Design review of the part built by this model. Coordinates are the model's own, in mm. Face numbers are marked on the shaded views. Coordinates: 2 decimals unless noted, no trailing zeros. Order: outer loops, then holes, each group sorted by start corner. A loop starts at its lowest first (then second) coordinate and runs counter-clockwise, first axis right, second up. Notation, with made-up numbers: M -16.5,12 L 6.5,12 A14 ccw 6.5,22 Z; hole C 67,6.5 d5. An arc over 180 degrees is marked long. Answer as a JSON object with one key per item and string values.
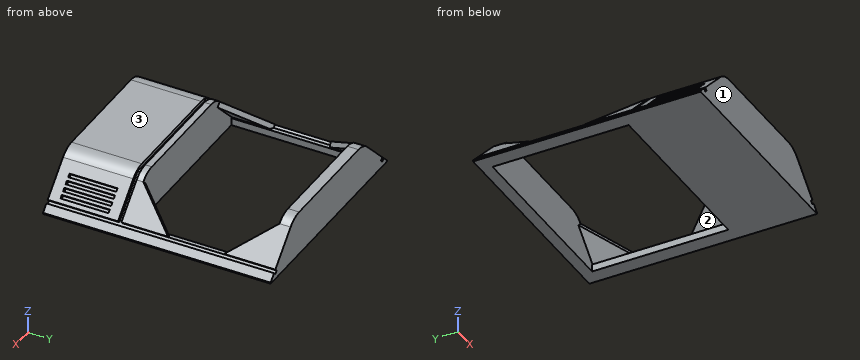
from build123d import *

# Parameters (mm, degrees)
F1_DEPTH  = 20.4
F3_DEPTH  = 0.3
F4_W      = 12.2
F4_H      = 3.3343145751
F5_DEPTH  = 8.8731825407
F6_W      = 8.2600505063
F6_H      = 12.2
F7_DEPTH  = 25
F8_W      = 4.3
F8_H      = 0.3
F9_DEPTH  = 0.3
F10_F1_R  = 2
F10_F2_R  = 2
F12_DEPTH = 0.5
F13_W     = 8.8721825407
F13_H     = 0.3
F14_DEPTH = 0.3
F16_DEPTH = 0.1


# Not quite as in the source:
# - a feature names something its author has since deleted; it is built from what else it names


with BuildPart() as f1:
    # F0 (on Front) → F1 (new body)
    with BuildSketch(Plane.XZ):
        Polygon((-9.65, 0), (0, 0), (0, 3.9), (-5.75, 3.9), align=None)
    extrude(amount=F1_DEPTH)

    # F2 (on face) → F3 (cut)
    with BuildSketch(Plane(origin=(-4.825, 0, 4.825), x_dir=(0, -1, 0), z_dir=(-0.7071067812, 0, 0.7071067812))):
        Polygon((13.8, -5.7235804385), (0, -5.7235804385), (0, -6.0235804385), (20.4, -6.0235804385), (20.4, -5.7235804385), (14.1, -5.7235804385), (14.1, 0.1956567054), (13.8, 0.1956567054), align=None)
    extrude(amount=-F3_DEPTH, mode=Mode.SUBTRACT)

    # F4 (on face) → F5 (cut, through all)
    with BuildSketch(Plane.YZ):
        with Locations((-7.1, 2.2328427125)):
            Rectangle(F4_W, F4_H)
    extrude(amount=-F5_DEPTH, mode=Mode.SUBTRACT)

    # F6 (on face) → F7 (cut)
    with BuildSketch(Plane.XY.offset(0.5656854249)):
        with Locations((-4.1300252532, -7.1)):
            Rectangle(F6_W, F6_H)
    extrude(amount=-F7_DEPTH, mode=Mode.SUBTRACT)

    # F8 (on face) → F9 (cut)
    with BuildSketch(Plane(origin=(-4.825, 0, 4.825), x_dir=(0, -1, 0), z_dir=(-0.7071067812, 0, 0.7071067812))):
        with Locations((17.25, -3.3735804385)):
            Rectangle(F8_W, F8_H)
        with Locations((17.25, -3.9735804385)):
            Rectangle(F8_W, F8_H)
        with Locations((17.25, -5.1735804385)):
            Rectangle(F8_W, F8_H)
        with Locations((17.25, -4.5735804385)):
            Rectangle(F8_W, F8_H)
    extrude(amount=-F9_DEPTH, mode=Mode.SUBTRACT)

    # F10: fillet of radius 2 on 3 edges, made by hand

    # F10_f1
    f10_f1_edges = [f1.edges().sort_by_distance(p)[0] for p in [
        (-5.75, -0.5, 3.9),
    ]]
    fillet(f10_f1_edges, radius=F10_F1_R)

    # F10_f2
    f10_f2_edges = [f1.edges().sort_by_distance(p)[0] for p in [
        (-5.75, -13.5, 3.9),
    ]]
    fillet(f10_f2_edges, radius=F10_F2_R)

    # F11 (on face) → F12 (join)
    with BuildSketch(Plane(origin=(-4.825, 0, 4.825), x_dir=(0, -1, 0), z_dir=(-0.7071067812, 0, 0.7071067812))):
        Polygon((1, -2.1365746699), (1, -5.7235804385), (4.5870057685, -5.7235804385), align=None)
        Polygon((13.2, -5.7235804385), (13.2, -2.1365746699), (9.6129942315, -5.7235804385), align=None)
    extrude(amount=-F12_DEPTH)

    # F13 (on face) → F14 (cut)
    with BuildSketch(Plane.XY.offset(3.9)):
        with Locations((-4.4360912703, -13.95)):
            Rectangle(F13_W, F13_H)
    extrude(amount=-F14_DEPTH, mode=Mode.SUBTRACT)

    # F15: F1 across face


with BuildPart() as f1_1:
    add(f1.part)
    add(f1.part.mirror(Plane(origin=(0, -16.8091639871, 1.9442122186), x_dir=(0, 1, 0), z_dir=(1, 0, 0))))

    # F16 (add): a face of the model
    f16_faces = [f1_1.faces().sort_by_distance(p)[0] for p in [
        (0, -13.4511563716, 0),
    ]]
    extrude(f16_faces, amount=F16_DEPTH)


solid = f1_1.part
1) Add section B-B (y = -6.25). State the section outline as (x, z) points, and give its area (3 significant figures).
Taken from the geometry:
{"outline": "M -9.65,-0.1 L -8.26,-0.1 L -8.26,0.57 L -8.66,0.57 L -8.87,0.35 L -9.08,0.57 L -9.65,0 Z; M 8.26,-0.1 L 9.65,-0.1 L 9.65,0 L 9.08,0.57 L 8.87,0.35 L 8.66,0.57 L 8.26,0.57 Z", "area": "1.44 mm2"}
2) To check wall thickness, follow L1, parallel to Y at x = 1.5, z = 1.6; L2, parallel to Z at x = 8.75, y = -4; L3, parallel to X at y = -11.5, z = 1. State the ranges of each line that lie inside material, in increasing order.
Taken from the geometry:
{"L1": "y = -20.4 to -13.2, -1 to 0", "L2": "z = -0.1 to 0.48, 0.66 to 0.9", "L3": "x = -8.65 to -7.94, 7.94 to 8.65"}
3) Add section C-C (y = -3.25). State the section outline as (x, z) points.
Taken from the geometry:
{"outline": "M -9.65,-0.1 L -8.26,-0.1 L -8.26,0.57 L -8.38,0.57 L -7.57,1.37 L -7.93,1.72 L -8.87,0.78 L -8.66,0.57 L -8.87,0.35 L -9.08,0.57 L -9.65,0 Z; M 7.57,1.37 L 8.38,0.57 L 8.26,0.57 L 8.26,-0.1 L 9.65,-0.1 L 9.65,0 L 9.08,0.57 L 8.87,0.35 L 8.66,0.57 L 8.87,0.78 L 7.93,1.72 Z"}
4) Mouldability with a two-part tool opening along Y and no side actions: class the marked faces 1, 2 and 3 as released by +Y, released by -Y, zero draft, split by the parting line, or undercut.
Taken from the geometry:
{"face 1": "released by -Y", "face 2": "undercut", "face 3": "zero draft"}
5) Add section A-A (x = 1.25). State the section outline as (y, z) points, and give its area (3 significant figures).
Taken from the geometry:
{"outline": "M -20.4,-0.1 L -13.2,-0.1 L -13.2,3.9 L -13.8,3.9 L -13.8,3.6 L -14.1,3.6 L -14.1,3.9 L -20.4,3.9 Z; M -1,-0.1 L 0,-0.1 L 0,3.9 L -1,3.9 Z", "area": "32.7 mm2"}
